from build123d import *

# Parameters (mm, degrees)
SKETCH1_W           = 30
SKETCH1_H           = 30
BOSS_EXTRUDE1_DEPTH = 7
SKETCH2_W           = 7
SKETCH2_H           = 30
BOSS_EXTRUDE2_DEPTH = 30
CUT_EXTRUDE1_DEPTH  = 30
SHELL1_T            = -1
BOSS_EXTRUDE3_DEPTH = 30
SHELL2_START        = 7
SHELL2_DEPTH        = 30


# Read off the part's stored shape, not the designer's step: Shell2
with BuildPart() as part:
    # Sketch1 → Boss-Extrude1 (new body)
    with BuildSketch(Plane.XY):
        with Locations((15, 15)):
            Rectangle(SKETCH1_W, SKETCH1_H)
    extrude(amount=BOSS_EXTRUDE1_DEPTH)

    # Sketch2 → Boss-Extrude2 (add)
    with BuildSketch(Plane.ZY):
        with Locations((3.5, 15)):
            Rectangle(SKETCH2_W, SKETCH2_H)
    extrude(amount=BOSS_EXTRUDE2_DEPTH)

    # Sketch3 → Cut-Extrude1 (cut)
    with BuildSketch(Plane.XY.offset(7)):
        Polygon((-30, 30), (0, 0), (-30, 0), align=None)
    extrude(amount=-CUT_EXTRUDE1_DEPTH, mode=Mode.SUBTRACT)

    # Shell1
    shell1_openings = [part.faces().sort_by_distance(p)[0] for p in [
        (0, 30, 3.5),
        (30, 15, 3.5),
    ]]
    offset(amount=SHELL1_T, openings=shell1_openings, kind=Kind.INTERSECTION)

    # Sketch6 → Boss-Extrude3 (add)
    with BuildSketch(Plane.XY.offset(7)):
        Polygon((0, 0), (4.949747468, 4.949747468), (-20.100505063, 30), (-30, 30), align=None)
    extrude(amount=BOSS_EXTRUDE3_DEPTH)

    # Shell2 outline → Shell2 (cut)
    with BuildSketch(Plane.XY.offset(SHELL2_START)):
        Polygon((-28.585786438, 30), (0, 1.414213562), (3.535533906, 4.949747468), (-21.514718626, 30), align=None)
    extrude(amount=SHELL2_DEPTH, mode=Mode.SUBTRACT)


solid = part.part
CAD build for the part. Positions are in the model's coordinates, mm. A direction names the side the tool comes from. Round coordinates to 2 decimals unless told otherwise and drop trailing zeros. Write each loop counter-clockwise with the first axis right and the second up, starting at its lowest first coordinate (ties: lowest second). Pieces come first, ordered by that corner, then holes. Notation, with made-up numbers: M 42,0.25 L 65,0.25 A15 cw 65,29.25 Z; hole C 57,68 d1. An arc over 180 degrees is marked long. Use a Markdown table: item, result. Add a question column.
1. Slice it at D-D on x = 2. Give the cut face in (y, z).
2. Flat gauge pins, fed straight in: P1, Ø15, axis at x = 14, y = 15, coming from the +Z side; P2, Ø6, axis at y = 23.5, z = 27.5, coming from the -X side; P3, Ø12, axis at x = 6, z = 32.5, coming from the +Y side. Where does each tip first touch, or does it go through?
3. Drill centre lines: probe 1 along Z at (x, y) = (22.5, 27); probe 2 along Z at (x, y) = (-8, 17.5); probe 3 along Y at (x, z) = (5.5, 2.5). Where is each one in solid material? Low to high.
4. Slice it at C-C on y = 11. Give the cut face in (x, z), then the cut area to 3 significant figures.
5. Pull direction X, two halves, no side cores. Call faces 5 (the face through (15, 1, 3)), 6 (the face through (2, 2, 22)), 7 (the face through (-8.814, 17.3, 21.79)): released by +X, released by -X, zero draft, split by the parting line, or undercut.
6. Slice it at B-B on x = 17.5. Give the cut face in (y, z), then the cut area to 3 significant figures.
7. Slice it at A-A on z = 10. Give the cut face in (x, y), then the cut area to 3 significant figures.
8. 3-axis set-ups, long thin cutter, end or side, ignore diameter. For faces 1 (the face through (-7.4, 17.3, 21.8)), 2 (the face through (8, 15, 1)), 3 (the face through (7, 15, 0)), 4 (the face through (-14.493, 15.907, 21.79)): which of +Z, -Z, +X, -X, +Y, -Y reach the whole face in a straight line?
Reply:
| question | item | result |
|---|---|---|
| 1 | outline | M 0,0 L 30,0 L 30,1 L 1,1 L 1,6 L 30,6 L 30,7 L 7.9,7 L 7.9,37 L 6.49,37 L 6.49,7 L 3.41,7 L 3.41,37 L 2,37 L 2,7 L 0,7 Z |
| 2 | P1 | stops at z = 7 |
| 2 | P2 | stops at x = -26.5 |
| 2 | P3 | stops at y = 9.9 |
| 3 | probe 1 | z = 0 to 1, 6 to 7 |
| 3 | probe 2 | z = 0 to 1, 6 to 37 |
| 3 | probe 3 | y = 0 to 1 |
| 4 | outline | M -11,0 L 30,0 L 30,1 L -9.59,1 L -9.59,6 L 30,6 L 30,7 L -1.1,7 L -1.1,37 L -2.51,37 L -2.51,7 L -9.59,7 L -9.59,37 L -11,37 Z |
| 4 | area | 174 mm^2 |
| 5 | face 5 | zero draft |
| 5 | face 6 | released by +X |
| 5 | face 7 | undercut |
| 6 | outline | M 0,0 L 30,0 L 30,1 L 1,1 L 1,6 L 30,6 L 30,7 L 0,7 Z |
| 6 | area | 65.0 mm^2 |
| 7 | outline | M -30,30 L 0,0 L 4.95,4.95 L -20.1,30 L -21.51,30 L 3.54,4.95 L 0,1.41 L -28.59,30 Z |
| 7 | area | 82.9 mm^2 |
| 8 | face 1 | +Z, +X, +Y |
| 8 | face 2 | +X, +Y |
| 8 | face 3 | -Z, +X, -X, +Y, -Y |
| 8 | face 4 | +Z |
